Design review of the part built by this model. Coordinates are the model's own, in mm. Face numbers are marked on the shaded views. A direction names the side the tool comes from. Coordinates: 2 decimals unless noted, no trailing zeros. Loops run counter-clockwise (first coordinate to the right, second up) from the corner with the lowest first, then second, coordinate; pieces in that order, holes last. Notation, with made-up numbers: (-27, 83) -> (11, 83) arc R30 cw to (11, 106) -> close; hole circle Ø1 at (14.25, 10). An arc over 180 degrees is marked (long way). Answer as a JSON object with one key per item and string values.
```python
from build123d import *

# Parameters (mm, degrees)
SKETCH005_R             = 2.25
SKETCH005_R_2           = 2
PAD003_DEPTH            = 2
SKETCH007_W             = 178
SKETCH007_H             = 109
SKETCH007_R             = 28.5
PAD005_DEPTH            = 54
SKETCH008_W             = 176.272423
SKETCH008_H             = 107.053562
POCKET001_DEPTH         = 48
BODY001_PLACEMENT_ANGLE = 180


with BuildPart() as part:
    # Sketch005 → Pad003 (new body)
    with BuildSketch(Plane.XY.offset(13)):
        with BuildLine():
            Line((-98.25, -54.5), (-98.25, 54.5))
            Line((-98.25, 54.5), (98.25, 54.5))
            Line((98.25, 54.5), (98.25, 48))
            Line((98.25, 48), (95.75, 48))
            ThreePointArc((95.75, 48), (93.75, 46), (95.75, 44))
            Line((95.75, 44), (98.25, 44))
            Line((98.25, 44), (98.25, -54.5))
            Line((98.25, -54.5), (-98.25, -54.5))
        make_face()
        with Locations((-93.25, -49.5)):
            Circle(SKETCH005_R, mode=Mode.SUBTRACT)
        with Locations((-35.75, 44.5)):
            Circle(SKETCH005_R_2, mode=Mode.SUBTRACT)
        with Locations((90.75, 44.5)):
            Circle(SKETCH005_R_2, mode=Mode.SUBTRACT)
        with Locations((90.75, -40.5)):
            Circle(SKETCH005_R_2, mode=Mode.SUBTRACT)
        with Locations((-35.75, -40.5)):
            Circle(SKETCH005_R_2, mode=Mode.SUBTRACT)
    extrude(amount=PAD003_DEPTH)

    # Sketch007 (on Face15 of Pad003) → Pad005 (join)
    with BuildSketch(Plane.XY.offset(15)):
        with Locations((9.36, 0)):
            Rectangle(SKETCH007_W, SKETCH007_H)
        with Locations((55.36, -11.5)):
            Circle(SKETCH007_R, mode=Mode.SUBTRACT)
    extrude(amount=PAD005_DEPTH)

    # Sketch008 (on Face5 of Pad005) → Pocket001 (cut)
    with BuildSketch(Plane.XY.offset(14)):
        with Locations((9.419559, -0.035154)):
            Rectangle(SKETCH008_W, SKETCH008_H)
    extrude(amount=POCKET001_DEPTH, mode=Mode.SUBTRACT)


with BuildPart() as part_1:
    # Body001 placement: moved
    add(part.part.moved(Location((-11.25, 0, -2))).rotate(Axis((-11.25, 0, -2), (0, 0, 1)), BODY001_PLACEMENT_ANGLE))


solid = part_1.part
```
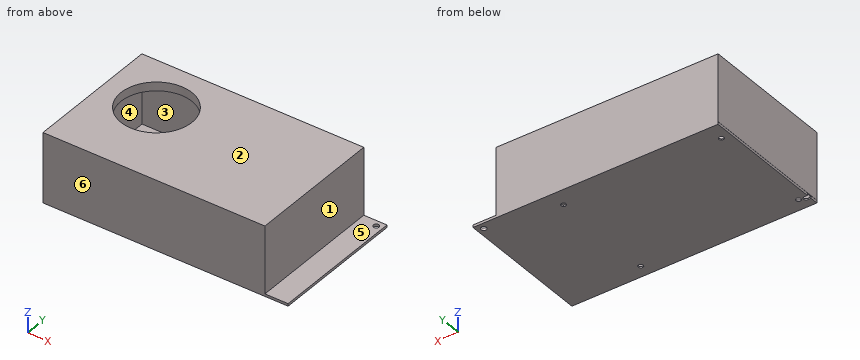
1) Wall thickness on probe 1 along Y at (x, z) = (82, 12.05); probe 2 along X at (y, z) = (11, 65); probe 3 along X at (y, z) = (32, 24.5): over which ranges is each line inside the solid? List them lowest first.
Completed:
{"probe 1": "-54.5 to 47.25, 51.75 to 54.5", "probe 2": "-109.61 to -95.11, -38.11 to 68.39", "probe 3": "-109.61 to -108.81, 67.47 to 68.39"}
2) Add section A-A, the plane y = 49.5. Give the boundary of the cut face in (x, z), and give its area (3 significant figures).
Completed:
{"outline": "(-109.61, 13) -> (-109.5, 13) -> (-109.5, 11) -> (79.75, 11) -> (79.75, 13) -> (68.39, 13) -> (68.39, 67) -> (-109.61, 67) -> close; (84.25, 11) -> (87, 11) -> (87, 13) -> (84.25, 13) -> close; hole (-108.81, 12) -> (67.47, 12) -> (67.47, 60) -> (-108.81, 60) -> close", "area": "1,530 mm²"}
3) The part is to be moulded in two halves that separate along X. For the marked faces 1, 2, 3 and 4, say which applies: pulls with the +X half, pulls with the -X half, needs draft (parallel to the pull), parting line crosses it, or undercut.
Completed:
{"face 1": "pulls with the +X half", "face 2": "needs draft", "face 3": "undercut", "face 4": "undercut"}
4) Clearance check with flat-ended pins moving along their axes: pin 1 Ø3 at (x, y) = (-102, 40.5) entering from -Z; pin 2 Ø1.5 at (y, z) = (0, 55.5) entering from +X; pin 3 Ø4 at (x, y) = (82, 49.5) entering from +Z; pin 4 Ø0.6 at (y, z) = (-18, 12.5) entering from -X. State where each tip first meets the part, or that it passes through.
Completed:
{"pin 1": "z = 60", "pin 2": "x = 68.39", "pin 3": "through", "pin 4": "x = -109.5"}
5) For the marked faces 5 and 6, list the 3-axis set-ups (+Z, -Z, +X, -X, +Y, -Y) from which the entire face can be reached by the end or side of a thin tool; tool diameter is ignored.
Completed:
{"face 5": "+Z, +X, +Y, -Y", "face 6": "+Z, -Z, +X, -X, -Y"}
6) Add section C-C, the plane y = -35. Give the boundary of the cut face in (x, z).
Completed:
{"outline": "(-109.61, 13) -> (-109.5, 13) -> (-109.5, 11) -> (87, 11) -> (87, 13) -> (68.39, 13) -> (68.39, 67) -> (-109.61, 67) -> close; hole (-108.81, 12) -> (67.47, 12) -> (67.47, 60) -> (-108.81, 60) -> close"}
7) Add section B-B, the plane x = 24.5. Give the boundary of the cut face in (y, z), and give its area (3 significant figures).
Completed:
{"outline": "(-54.5, 11) -> (-46.5, 11) -> (-46.5, 12) -> (-53.49, 12) -> (-53.49, 60) -> (53.56, 60) -> (53.56, 12) -> (42.5, 12) -> (42.5, 11) -> (54.5, 11) -> (54.5, 67) -> (-54.5, 67) -> close; (-42.5, 11) -> (38.5, 11) -> (38.5, 12) -> (-42.5, 12) -> close", "area": "957 mm²"}
8) Add section D-D, the plane z = 32.5. Give the boundary of the cut face in (x, y), and give its area (3 significant figures).
Completed:
{"outline": "(-109.61, -54.5) -> (68.39, -54.5) -> (68.39, 54.5) -> (-109.61, 54.5) -> close; hole (-108.81, -53.49) -> (67.47, -53.49) -> (67.47, 53.56) -> (-108.81, 53.56) -> close", "area": "531 mm²"}
